Geometry: final body of the model. Coordinates: model frame, mm. Face numbers are marked on the shaded views. Give positions to 0.01 mm unless a question says otherwise; leave off trailing zeros. Write each loop counter-clockwise with the first axis right and the second up, starting at its lowest first coordinate (ties: lowest second). Pieces come first, ordered by that corner, then holes.
Q1. Section B-B (y = -6.75). Return the cut outline in (x, z).
Q2. Section C-C (y = -12.75). Return the cut outline in (x, z), plus the area to 3 significant figures.
Q3. Section A-A (x = -23.5). Return the cut outline in (y, z), plus the area to 3 significant figures.
Q4. Pin query (flat end, axial travel): pin 1 Ø3.5 at (x, z) = (-15.43, 0) entering from -Y; pin 2 Ø1.8 at (x, y) = (-34, -7) entering from +Z. Return the tip coordinate at first contact, or that it passes through.
Q5. Line query: line 1 (X direction, y = -3, z = 0); line 2 (X direction, y = -0.75, z = -1); line 3 (Y direction, x = -7, z = 2.5). Output: solid intervals per line, ascending.
Q6. Mould query, pull axis X, two halves, no side actions, for the marked faces 1, 2 and 3. Classes: +X half, -X half, draft (parallel to the pull), parting line (faces both ways), or undercut.
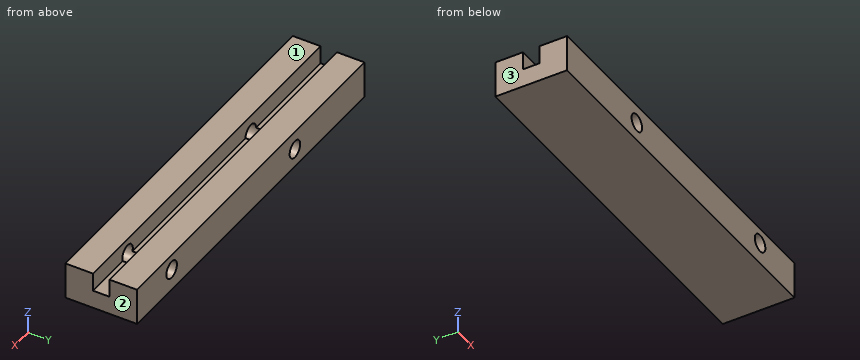
from build123d import *

# Parameters (mm, degrees)
F0_W     = 79.679102
F0_H     = 7.809082
F1_DEPTH = 15.24
F2_W     = 3.50939
F2_H     = 3.868172
F3_DEPTH = 63.5
F4_R     = 1.8415
F5_DEPTH = 32.7406


with BuildPart() as f1:
    # F0 (on Front) → F1 (new body)
    with BuildSketch(Plane.XZ):
        Rectangle(F0_W, F0_H)
    extrude(amount=F1_DEPTH)

    # F2 (on Right) → F3 (cut, symmetric)
    with BuildSketch(Plane.YZ):
        with Locations((-7.615543, 5.802258)):
            Rectangle(F2_W, F2_H)
        with Locations((-7.615543, 1.934086)):
            Rectangle(F2_W, F2_H)
    extrude(amount=F3_DEPTH, both=True, mode=Mode.SUBTRACT)

    # F4 (on face) → F5 (cut)
    with BuildSketch(Plane(origin=(0, 0, 0), x_dir=(-1, 0, 0), z_dir=(0, 1, 0))):
        with Locations((-27.754245, 0.657367)):
            Circle(F4_R)
        with Locations((15.429531, 0)):
            Circle(F4_R)
    extrude(amount=-F5_DEPTH, mode=Mode.SUBTRACT)


solid = f1.part
Computed:
1. outline: (-39.84, -3.9) - (39.84, -3.9) - (39.84, 0) - (29.47, 0) arc R1.84 cw to (26.03, 0) - (-13.59, 0) arc R1.84 cw to (-17.27, 0) - (-39.84, 0) - close
2. outline: (-39.84, -3.9) - (39.84, -3.9) - (39.84, 3.9) - (-39.84, 3.9) - close; hole circle Ø3.68 at (-15.43, 0); hole circle Ø3.68 at (27.75, 0.66)
2. area: 601 mm2
3. outline: (-15.24, -3.9) - (0, -3.9) - (0, 3.9) - (-5.86, 3.9) - (-5.86, 0) - (-9.37, 0) - (-9.37, 3.9) - (-15.24, 3.9) - close
3. area: 105 mm2
4. pin 1: passes through
4. pin 2: stops at z = 0
5. line 1: x = -39.84 to -17.27, -13.59 to 26.03, 29.47 to 39.84
5. line 2: x = -39.84 to -16.98, -13.88 to 26.95, 28.56 to 39.84
5. line 3: y = -15.24 to -9.37, -5.86 to 0
6. face 1: draft
6. face 2: +X half
6. face 3: -X half
